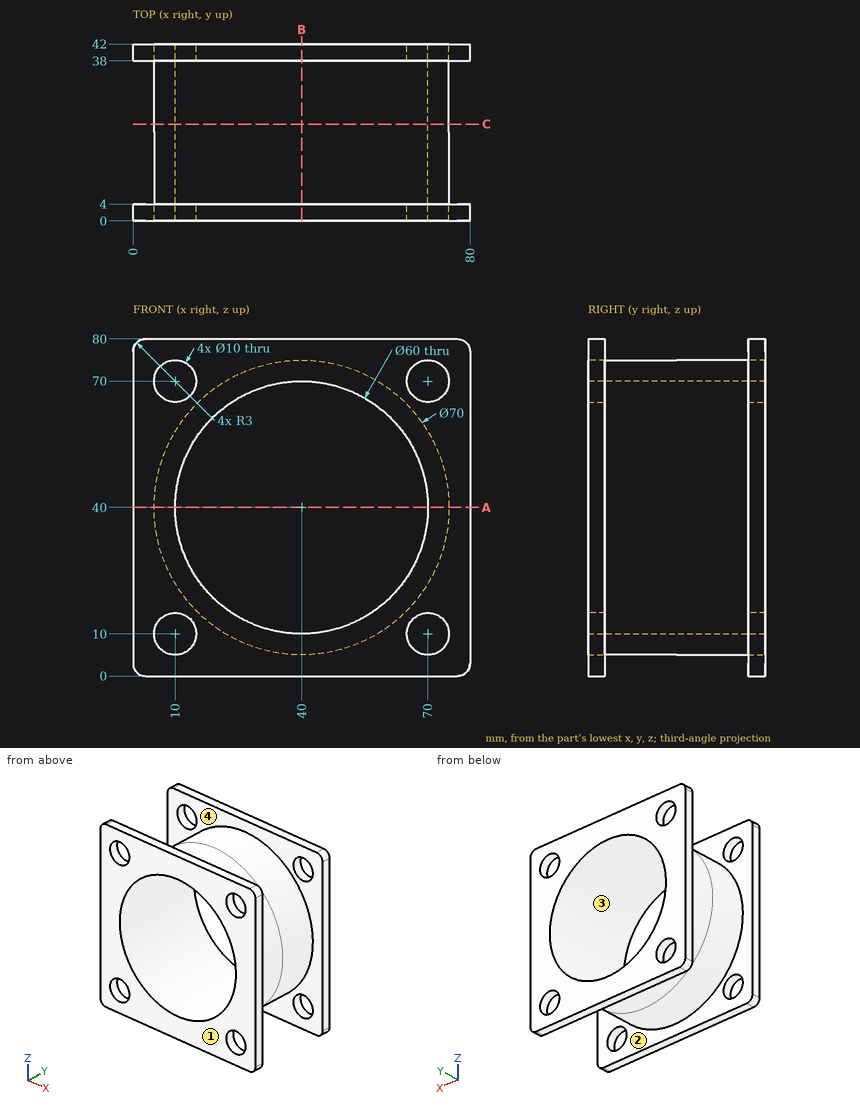
Could you check a few things on this drawing? It's one solid part, dimensions in mm from its lowest x, y, z. A direction names the side the tool comes from. Give positions to 0.01 mm unless a question says otherwise; leave off trailing zeros. Order: outer loops, then holes, each group sorted by start corner. A loop starts at its lowest first (then second) coordinate and runs counter-clockwise, first axis right, second up. Notation, with made-up numbers: M 50.25,87.5 L 81.25,87.5 A32 cw 81.25,123.5 Z; hole C 7,62.25 d8. An arc over 180 degrees is marked long. Use one line per item in the form item = value. Start each with the question number.
Item 1: If we section it at A-A (z = 40): Write out the boundary of the cut face in (x, y), then the cut area to 3 significant figures.
Item 2: If we section it at B-B (x = 40): Write out the boundary of the cut face in (y, z), then the cut area to 3 significant figures.
Item 3: If we section it at C-C (y = 23): Write out the boundary of the cut face in (x, z).
Item 4: Will these pins go through, and if not, where does the flat tip stop? pin 1 Ø8 at (y, z) = (31.5, 22.5) entering from -X; pin 2 Ø8 at (x, z) = (70, 10) entering from -Y; pin 3 Ø10 at (x, y) = (42.5, 27.5) entering from -Z; pin 4 Ø4 at (y, z) = (24, 21) entering from +X.
Item 5: For the marked faces 1 and 2, which set-ups out of +Z, -Z, +X, -X, +Y, -Y let a thin tool reach every point of the face, with its end or its side?
Item 6: If I drill on line 1 along Y through (x, z) = (69, 18.5); line 2 along Z through (x, y) = (40.5, 7), over which ranges is the centre line in solid material (lowest first)?
Item 7: We'd pull the mould along X, two halves only. Please class the marked faces 3 and 4: +X half, -X half, draft (parallel to the pull), parting line (faces both ways), or undercut.
Outcome:
q1.outline = M 0,0 L 10,0 L 10,42 L 0,42 L 0,38 L 5,38 L 5,4 L 0,4 Z; M 70,0 L 80,0 L 80,4 L 75,4 L 75,38 L 80,38 L 80,42 L 70,42 Z
q1.area = 500 mm2
q2.outline = M 0,0 L 4,0 L 4,5 L 38,5 L 38,0 L 42,0 L 42,10 L 0,10 Z; M 0,70 L 42,70 L 42,80 L 38,80 L 38,75 L 4,75 L 4,80 L 0,80 Z
q2.area = 500 mm2
q3.outline = C 40,40 d70; hole C 40,40 d60
q4.pin_1 = 7.71
q4.pin_2 = through
q4.pin_3 = 5
q4.pin_4 = 70.59
q5.face_1 = +Z, -Z, +X, -X, -Y
q5.face_2 = none
q6.line_1 = 0 to 4, 38 to 42
q6.line_2 = 5 to 10, 70 to 75
q7.face_3 = undercut
q7.face_4 = draft
